Autodesk Inventor part; units mm, degrees
ref_plane "YZ Plane" through (0, 0, 0) normal (1, 0, 0) x (0, 1, 0)
ref_plane "XZ Plane" through (0, 0, 0) normal (0, 1, 0) x (-1, 0, 0)
ref_plane "XY Plane" through (0, 0, 0) normal (0, 0, 1) x (1, 0, 0)
sketch "Skizze1" plane through (0, 0, 0) normal (0, 0, 1) x (1, 0, 0)
  line L0 (0, 0) -> (-100, 0)
  line L1 (-100, 0) -> (-100, 40)
  line L2 (-100, 40) -> (0, 40)
  line L3 (0, 40) -> (0, 0)
  dimension "d0" = 100
  dimension "d1" = 40
extrude "Extrusion1" add sketch "Skizze1" along normal blind 15
sketch "Skizze2" plane through (0, 0, 15) normal (0, 0, 1) x (1, 0, 0)
  line L0 (-100, 40) -> (-100, 0)
  line L1 (-100, 25) -> (0, 25)
  line L2 (0, 25) -> (0, 15)
  line L3 (0, 15) -> (-100, 15)
  line L4 (-100, 15) -> (-100, 25)
  line L5 (0, 40) -> (-100, 40)
  line L6 (-100, 0) -> (0, 0)
  line L7 (0, 0) -> (0, 40)
  dimension "d4" = 15
  dimension "d5" = 15
extrude "Extrusion2" cut sketch "Skizze2" against normal blind 9 contours L1 L2 L3 L0
sketch "Skizze3" plane through (0, 0, 15) normal (0, 0, 1) x (1, 0, 0)
  line L0 (0, 0) -> (0, 15)
  line L1 (-100, 0) -> (0, 0)
  line L2 (-100, 25) -> (0, 25)
  point P0 (-5, 32.5)
  point P1 (-80.5, 32.5)
  point P2 (-5, 7.5)
  point P3 (-80.5, 7.5)
  dimension "d8" = 75.5
  dimension "d9" = 5
  dimension "d10" = 7.5
  dimension "d11" = 7.5
hole "Bohrung1" at (-5, 32.5, 15) at (-80.5, 32.5, 15) at (-5, 7.5, 15) at (-80.5, 7.5, 15) direction (0, 0, -1) diameter 3.6 end through all
sketch "Skizze4" plane through (0, 0, 6) normal (0, 0, 1) x (1, 0, 0)
  line L0 (-100, 15) -> (-100, 25)
  line L1 (0, 15) -> (-100, 15)
  point P0 (0, 0)
  point P1 (-10, 20)
  point P2 (-90, 20)
  dimension "d19" = 80
  dimension "d20" = 10
  dimension "d21" = 5
hole "Bohrung2" at (-10, 20, 6) at (-90, 20, 6) direction (0, 0, -1) diameter 5.8 end through all counterbore diameter 15 counterbore depth 1
hole "Bohrung3" at (-10, 20, 6) at (-90, 20, 6) direction (0, 0, 1) diameter 15 end through all
chamfer "Fase1" distance 3 angle 45 2 edges at (-50, 0, 15) (-50, 40, 15)
chamfer "Fase2" distance 1.25 angle 45 6 edges at (-97.7951, 25, 15) (-2.2049, 25, 15) (-50, 25, 15) (-97.7951, 15, 15) (-2.2049, 15, 15) (-50, 15, 15)
properties part number "pcb_x_carriage_addon"
CAD build for the part. Positions are in the model's coordinates, mm. A direction names the side the tool comes from. Coordinates: 2 decimals unless noted, no trailing zeros. Write each loop counter-clockwise with the first axis right and the second up, starting at its lowest first coordinate (ties: lowest second). Pieces come first, ordered by that corner, then holes. Notation, with made-up numbers: M -32.5,1 L -2.5,1 A23 ccw -2.5,25 Z; hole C 25,27.25 d2. An arc over 180 degrees is marked long. Answer as a JSON object with one key per item and string values. Group by question number.
1) Tool access for faces 1 (the face through (-2, 25, 10)), 2 (the face through (-100, 19.7, 5.7)): list every direction of +Z, -Z, +X, -X, +Y, -Y with a clear straight run to the whole face (end or side of a thin tool).
2) Pin check, flat tips, straight feed: pin 1 Ø3 at (x, y) = (-50.5, 19.5) entering from +Z; pin 2 Ø1.5 at (x, z) = (-37, 13.5) entering from -Y; pin 3 Ø3.5 at (x, y) = (-10, 20) entering from +Z. Stop position of each tip, or through.
3) Saw through at C-C (x = -80.5). Write the cut outline in (y, z), plus the area to 3 significant figures.
4) Mould opens along Y. For faces 3 (the face through (-98, 25, 10)), 4 (the face through (-49, 0, 6)), 5 (the face through (-90.1, 16.8, 5)), 6 (the face through (0, 20.3, 5.7)) say: +Y half, -Y half, draft (parallel to the pull), parting line (faces both ways), or undercut.
5) Saw through at D-D (z = 3). Write the cut outline in (x, y).
6) Wall check: line 1 (X direction, y = 20, z = 1.85); line 2 (X direction, y = 32.5, z = 14.5); line 3 (Y direction, x = -82.5, z = 8.5). Give the ranges that are in metal, low to high. Write a range as from..to.
7) Saw through at A-A (z = 8). Write the cut outline in (x, y).
8) Saw through at B-B (y = 20). Write the cut outline in (x, z).
Values follow:
{
 "1": {"face 1": "+Z, +X, -X", "face 2": "+Z, -Z, -X, +Y, -Y"},
 "2": {"pin 1": "stops at z = 6", "pin 2": "stops at y = 0.75", "pin 3": "passes through"},
 "3": {"outline": "M 0,0 L 5.7,0 L 5.7,15 L 3,15 L 0,12 Z; M 9.3,0 L 30.7,0 L 30.7,15 L 26.25,15 L 25,13.75 L 25,6 L 15,6 L 15,13.75 L 13.75,15 L 9.3,15 Z; M 34.3,0 L 40,0 L 40,12 L 37,15 L 34.3,15 Z", "area": "391 mm2"},
 "4": {"face 3": "undercut", "face 4": "-Y half", "face 5": "undercut", "face 6": "draft"},
 "5": {"outline": "M -100,0 L 0,0 L 0,40 L -100,40 Z; hole C -90,20 d5.8; hole C -80.5,7.5 d3.6; hole C -80.5,32.5 d3.6; hole C -10,20 d5.8; hole C -5,7.5 d3.6; hole C -5,32.5 d3.6"},
 "6": {"line 1": "x = -100..-92.9, -87.1..-12.9, -7.1..0", "line 2": "x = -100..-82.3, -78.7..-6.8, -3.2..0", "line 3": "y = 0..15, 25..40"},
 "7": {"outline": "M -100,0 L 0,0 L 0,15 L -4.41,15 A7.5 cw -15.59,15 L -84.41,15 A7.5 cw -95.59,15 L -100,15 Z; M -100,25 L -95.59,25 A7.5 cw -84.41,25 L -15.59,25 A7.5 cw -4.41,25 L 0,25 L 0,40 L -100,40 Z; hole C -80.5,7.5 d3.6; hole C -80.5,32.5 d3.6; hole C -5,7.5 d3.6; hole C -5,32.5 d3.6"},
 "8": {"outline": "M -100,0 L -92.9,0 L -92.9,5 L -97.5,5 L -97.5,6 L -100,6 Z; M -87.1,0 L -12.9,0 L -12.9,5 L -17.5,5 L -17.5,6 L -82.5,6 L -82.5,5 L -87.1,5 Z; M -7.1,0 L 0,0 L 0,6 L -2.5,6 L -2.5,5 L -7.1,5 Z"}
}
